Job drawing, mm, ordinate dimensions from the low corner. One solid piece. A direction names the side the tool comes from. Round coordinates to 2 decimals unless told otherwise and drop trailing zeros. Order: outer loops, then holes, each group sorted by start corner. A loop starts at its lowest first (then second) coordinate and runs counter-clockwise, first axis right, second up. Notation, with made-up numbers: (-37, 70) - (16, 70) arc R22 ccw to (16, 82) - close; hole circle Ø1 at (56.5, 79.25). An arc over 180 degrees is marked (long way). Write each question's results on one line, items separated by ' | '. Start each with the question number.
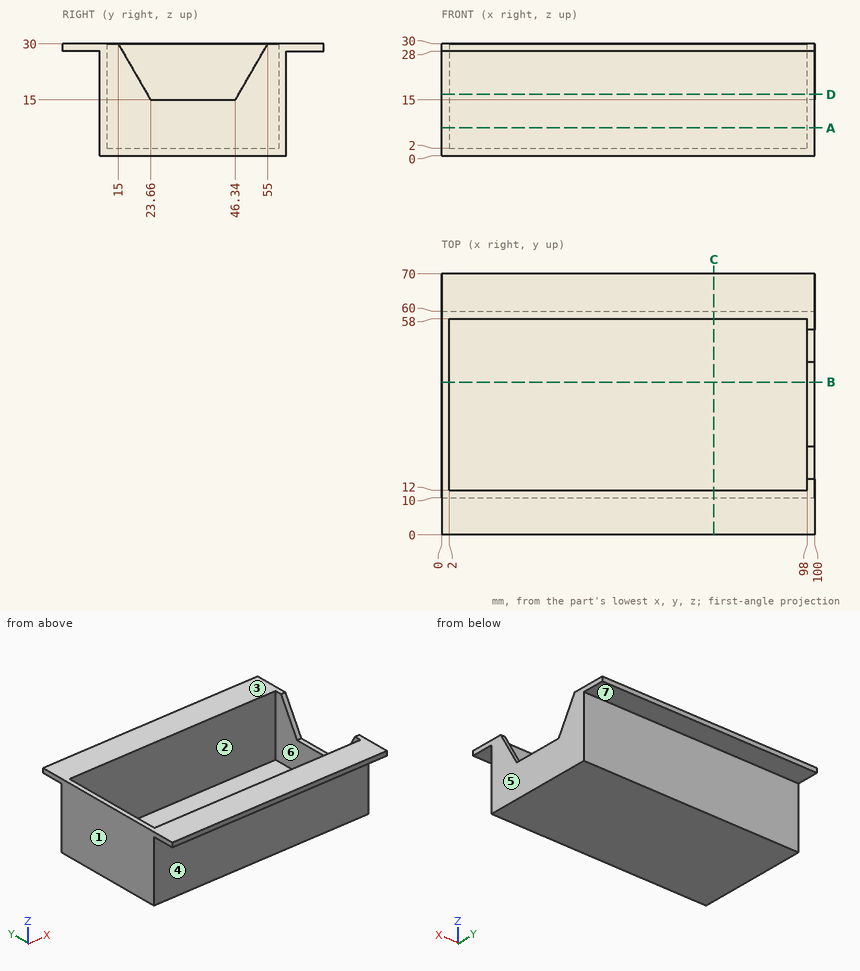
1. Wall check: line 1 (Y direction, x = 53, z = 21.75); line 2 (Y direction, x = 54, z = 28.25); line 3 (X direction, y = 46, z = 9). Give the ranges that are in metal, low to high. Write a range as from..to.
2. Cut at D-D (z = 16.5). List the corners of the cut face in (x, y).
3. Cut at C-C (x = 73). List the corners of the cut face in (y, z), plus the area to 3 significant figures.
4. Mould opens along X. For the marked faces 1, 2 and 3 say: pulls with the +X half, pulls with the -X half, needs draft (parallel to the pull), parting line crosses it, or undercut.
5. 3-axis set-ups, long thin cutter, end or side, ignore diameter. For the marked faces 4, 5, 6 and 7: which of +Z, -Z, +X, -X, +Y, -Y reach the whole face in a straight line?
6. Flat gauge pins, fed straight in: pin 1 Ø3 at (x, y) = (49.5, 64.5) entering from -Z; pin 2 Ø8.5 at (x, z) = (68, 9) entering from +Y; pin 3 Ø23 at (x, y) = (28, 36) entering from +Z. Where does each tip first touch, or does it go through?
7. Cut at A-A (z = 7.5). List the corners of the cut face in (x, y), plus the area to 3 significant figures.
8. Cut at B-B (y = 41). List the corners of the cut face in (x, z).
A:
1) line 1: y = 10..12, 58..60 | line 2: y = 0..12, 58..70 | line 3: x = 0..2, 98..100
2) outline: (0, 10) - (100, 10) - (100, 22.79) - (98, 22.79) - (98, 12) - (2, 12) - (2, 58) - (98, 58) - (98, 47.21) - (100, 47.21) - (100, 60) - (0, 60) - close
3) outline: (0, 28) - (10, 28) - (10, 0) - (60, 0) - (60, 28) - (70, 28) - (70, 30) - (58, 30) - (58, 2) - (12, 2) - (12, 30) - (0, 30) - close | area: 252 mm^2
4) face 1: pulls with the -X half | face 2: undercut | face 3: needs draft
5) face 4: -Z, +X, -X, -Y | face 5: +Z, -Z, +X, +Y, -Y | face 6: +Z | face 7: -Z, +X, -X, +Y
6) pin 1: stops at z = 28 | pin 2: stops at y = 60 | pin 3: stops at z = 2
7) outline: (0, 10) - (100, 10) - (100, 60) - (0, 60) - close; hole (2, 12) - (98, 12) - (98, 58) - (2, 58) - close | area: 584 mm^2
8) outline: (0, 0) - (100, 0) - (100, 15) - (98, 15) - (98, 2) - (2, 2) - (2, 30) - (0, 30) - close
